from build123d import *

# Parameters (mm, degrees)
SKETCH_1_W                                     = 30.8
SKETCH_1_H                                     = 12.55
M3_01_THINFLANGE_30_80X12_55X0_60_DEPTH        = 0.6
SKETCH_2_W                                     = 30.8
SKETCH_2_H                                     = 12.55
M3_02_FIRSTSHOULDER_30_80X12_55_D7_00_DEPTH    = 7
SKETCH_3_W                                     = 20
SKETCH_3_H                                     = 14
M3_03_SECONDSTAGECORE_20_00X14_00_D22_00_DEPTH = 22
SKETCH_4_R                                     = 2.5
M3_04_SIMPLIFIEDFIXEDPOSTS_DIA5_00_L3_50_DEPTH = 3.5
M3_05_ROUNDEDDGUIDE_OUTERBOSS_L4_00_DEPTH      = 4
M3_06_ROUNDEDDGUIDE_INNEROPENING_DEPTH         = 4
SKETCH_7_R                                     = 0.5
M3_07_9PINS_DIA1_00_L4_00_DEPTH                = 4
SKETCH_8_R                                     = 1.6
M3_08_FIXEDPOSTBORES_DIA3_20_PITCH25_00_DEPTH  = 4


with BuildPart() as part:
    # 草图1 → M3_01_ThinFlange_30.80x12.55x0.60 (new body)
    with BuildSketch(Plane.XY):
        Rectangle(SKETCH_1_W, SKETCH_1_H)
    extrude(amount=-M3_01_THINFLANGE_30_80X12_55X0_60_DEPTH)

    # 草图2 → M3_02_FirstShoulder_30.80x12.55_D7.00 (add)
    with BuildSketch(Plane.XY):
        Rectangle(SKETCH_2_W, SKETCH_2_H)
    extrude(amount=-M3_02_FIRSTSHOULDER_30_80X12_55_D7_00_DEPTH)

    # 草图3 → M3_03_SecondStageCore_20.00x14.00_D22.00_FromFlange (add)
    with BuildSketch(Plane.XY):
        Rectangle(SKETCH_3_W, SKETCH_3_H)
    extrude(amount=-M3_03_SECONDSTAGECORE_20_00X14_00_D22_00_DEPTH)

    # 草图4 → M3_04_SimplifiedFixedPosts_Dia5.00_L3.50 (add)
    with BuildSketch(Plane.XY):
        with Locations((-12.5, 0)):
            Circle(SKETCH_4_R)
        with Locations((12.5, 0)):
            Circle(SKETCH_4_R)
    extrude(amount=-M3_04_SIMPLIFIEDFIXEDPOSTS_DIA5_00_L3_50_DEPTH)

    # 草图5 → M3_05_RoundedDGuide_OuterBoss_L4.00 (add)
    with BuildSketch(Plane.XY):
        with BuildLine():
            Line((-7.478140403, 4.15), (7.478140403, 4.15))
            ThreePointArc((7.478140403, 4.15), (8.071894431, 3.858209727), (8.20364406, 3.209883078))
            Line((8.20364406, 3.209883078), (6.421716349, -3.590116922))
            ThreePointArc((6.421716349, -3.590116922), (6.154422419, -3.993754028), (5.696212692, -4.15))
            Line((5.696212692, -4.15), (-5.696212692, -4.15))
            ThreePointArc((-5.696212692, -4.15), (-6.154422419, -3.993754028), (-6.421716349, -3.590116922))
            Line((-6.421716349, -3.590116922), (-8.20364406, 3.209883078))
            ThreePointArc((-8.20364406, 3.209883078), (-8.071894431, 3.858209727), (-7.478140403, 4.15))
        make_face()
    extrude(amount=M3_05_ROUNDEDDGUIDE_OUTERBOSS_L4_00_DEPTH)

    # 草图6 → M3_06_RoundedDGuide_InnerOpening (cut)
    with BuildSketch(Plane.XY):
        with BuildLine():
            Line((-6.999952877, 3.45), (6.999952877, 3.45))
            ThreePointArc((6.999952877, 3.45), (7.443485369, 3.225236726), (7.524509443, 2.734650647))
            Line((7.524509443, 2.734650647), (5.696248574, -3.065349353))
            ThreePointArc((5.696248574, -3.065349353), (5.496928733, -3.343532493), (5.171692007, -3.45))
            Line((5.171692007, -3.45), (-5.171692007, -3.45))
            ThreePointArc((-5.171692007, -3.45), (-5.496928733, -3.343532493), (-5.696248574, -3.065349353))
            Line((-5.696248574, -3.065349353), (-7.524509443, 2.734650647))
            ThreePointArc((-7.524509443, 2.734650647), (-7.443485369, 3.225236726), (-6.999952877, 3.45))
        make_face()
    extrude(amount=M3_06_ROUNDEDDGUIDE_INNEROPENING_DEPTH, mode=Mode.SUBTRACT)

    # 草图7 → M3_07_9Pins_Dia1.00_L4.00 (add)
    with BuildSketch(Plane.XY):
        with Locations(Location((-5.54, 1.42, 0), (0, 0, 180))):
            Circle(SKETCH_7_R)
        with Locations(Location((-2.77, 1.42, 0), (0, 0, 180))):
            Circle(SKETCH_7_R)
        with Locations(Location((0, 1.42, 0), (0, 0, 180))):
            Circle(SKETCH_7_R)
        with Locations(Location((2.77, 1.42, 0), (0, 0, 180))):
            Circle(SKETCH_7_R)
        with Locations(Location((5.54, 1.42, 0), (0, 0, 180))):
            Circle(SKETCH_7_R)
        with Locations(Location((-4.155, -1.42, 0), (0, 0, 180))):
            Circle(SKETCH_7_R)
        with Locations(Location((-1.385, -1.42, 0), (0, 0, 180))):
            Circle(SKETCH_7_R)
        with Locations(Location((1.385, -1.42, 0), (0, 0, 180))):
            Circle(SKETCH_7_R)
        with Locations(Location((4.155, -1.42, 0), (0, 0, 180))):
            Circle(SKETCH_7_R)
    extrude(amount=M3_07_9PINS_DIA1_00_L4_00_DEPTH)

    # 草图8 → M3_08_FixedPostBores_Dia3.20_Pitch25.00 (cut)
    with BuildSketch(Plane.XY):
        with Locations((-12.5, 0)):
            Circle(SKETCH_8_R)
        with Locations((12.5, 0)):
            Circle(SKETCH_8_R)
    extrude(amount=-M3_08_FIXEDPOSTBORES_DIA3_20_PITCH25_00_DEPTH, mode=Mode.SUBTRACT)


solid = part.part
Geometry: final body of the model. Coordinates: model frame, mm. A direction names the side the tool comes from. Round coordinates to 2 decimals unless told otherwise and drop trailing zeros. Order: outer loops, then holes, each group sorted by start corner. A loop starts at its lowest first (then second) coordinate and runs counter-clockwise, first axis right, second up.
Q1. Section D-D, the plane z = -3. Output: boundary loops of the cut face in (x, y) (3 decimals).
Result sheet:
outline: (-15.4, -6.275) - (-10, -6.275) - (-10, -7) - (10, -7) - (10, -6.275) - (15.4, -6.275) - (15.4, 6.275) - (10, 6.275) - (10, 7) - (-10, 7) - (-10, 6.275) - (-15.4, 6.275) - close; hole circle Ø3.2 at (-12.5, 0); hole circle Ø3.2 at (12.5, 0)
Q2. Access query for faces 1 (the face through (0, -4.15, 2)), 2 (the face through (-13, -6.275, -3)), 3 (the face through (-14.1, 0.07, -1.97)), 4 (the face through (0, 7, -11)), 5 (the face through (13, -6.275, -3)). Directions: +Z, -Z, +X, -X, +Y, -Y. A direction counts if a zero-diameter tool reaches every point of the face in a straight line with its end or side. Return the directions, or none.
Result sheet:
face 1: +Z, +X, -X, -Y
face 2: +Z, -Z, -X, -Y
face 3: +Z
face 4: +Z, -Z, +X, -X, +Y
face 5: +Z, -Z, +X, -Y
Q3. Section B-B, the plane x = -2.77. Output: boundary loops of the cut face in (y, z), and give its area (3 significant figures).
Result sheet:
outline: (-7, -22) - (7, -22) - (7, 0) - (4.15, 0) - (4.15, 4) - (3.45, 4) - (3.45, 0) - (1.92, 0) - (1.92, 4) - (0.92, 4) - (0.92, 0) - (-3.45, 0) - (-3.45, 4) - (-4.15, 4) - (-4.15, 0) - (-7, 0) - close
area: 318 mm2
Q4. Material intervals for probe 1 along Y at (x, z) = (5, 2); probe 2 along Y at (x, z) = (12.5, -1.8) (3 decimals); probe 3 along Z at (x, y) = (-13.5, -4.75), sorted ascending.
Result sheet:
probe 1: y = -4.15 to -3.45, 3.45 to 4.15
probe 2: y = -6.275 to -1.6, 1.6 to 6.275
probe 3: z = -7 to 0
Q5. Mould query, pull axis Y, two halves, no side actions, for faces 6 (the face through (0, 4, 4)), 7 (the face through (0, 4.15, 2)), 8 (the face through (2.308, 1.612, 1.972)). Classes: released by +Y, released by -Y, zero draft, split by the parting line, or undercut.
Result sheet:
face 6: zero draft
face 7: released by +Y
face 8: undercut
Q6. Pin query (flat end, axial travel): pin 1 (2.5 mm diameter, centred on x = 12, y = -0.5, fed in from +Z); pin 2 (2.5 mm diameter, centred on x = 12.5, y = 0, fed in from +Z); pin 3 (2.5 mm diameter, centred on x = 13.5, y = 0.5, fed in from -Z). Return the tip coordinate at first contact, or that it passes through.
Result sheet:
pin 1: stops at z = 0
pin 2: stops at z = -4
pin 3: stops at z = -7
Q7. Section C-C, the plane y = -5.25. Output: boundary loops of the cut face in (x, z).
Result sheet:
outline: (-15.4, -7) - (-10, -7) - (-10, -22) - (10, -22) - (10, -7) - (15.4, -7) - (15.4, 0) - (-15.4, 0) - close
Q8. Section A-A, the plane z = 0.5. Give the number of separate pieces and of enclosed holes in the cut face, and give its area (3 significant figures).
Result sheet:
separate pieces: 10
enclosed holes: 1
area: 37.1 mm2
